from build123d import *

# Parameters (mm, degrees)
F0_W     = 46
F0_H     = 43
F0_R     = 2.5
F1_DEPTH = 3.5
F2_R     = 0.5


with BuildPart() as f1:
    # F0 (on Top) → F1 (new body)
    with BuildSketch(Plane.XY):
        with Locations((-3.022213, -8.843659)):
            Rectangle(F0_W, F0_H)
        with Locations((-3.022213, -12.343659)):
            Circle(F0_R, mode=Mode.SUBTRACT)
    extrude(amount=F1_DEPTH)

    # F2
    f2_edges = [f1.edges().sort_by_distance(p)[0] for p in [
        (-3.022213, 12.656341, 3.5),
        (-26.022213, -8.843659, 3.5),
        (-3.022213, -30.343659, 3.5),
        (19.977787, -8.843659, 3.5),
        (-5.522213, -12.343659, 3.5),
    ]]
    fillet(f2_edges, radius=F2_R)


solid = f1.part
Verification items for the finished model (mm, model axes). Give positions to 0.01 mm unless a question says otherwise; leave off trailing zeros.
1) Thickness scan on line 1 along Y through (x, z) = (-5, 3.3); line 2 along X through (y, z) = (-13.5, 2.9); line 3 along X through (y, z) = (-14.5, 2). Record the ranges inside material, lowest first.
2) Depth check by flat-ended pin: pin 1 Ø8 at (x, y) = (-9, -12.5) entering from -Z. Enter the tip coordinate at first touch or a pass-through.
3) Draft check along X on faces 1 (the flat face through (-3, -9, 0)), 2 (the cylindrical face through (-3.564, -14.784, 1.479)), 3 (the flat face through (-26.022, -9, 1)). Enter one of: pulls with the +X half, pulls with the -X half, needs draft (parallel to the pull), parting line crosses it, or undercut.
Answers:
1. line 1: y = -30.24 to -14.03, -10.66 to 12.56
1. line 2: x = -26.02 to -5.24, -0.81 to 19.98
1. line 3: x = -26.02 to -4.29, -1.76 to 19.98
2. pin 1: stops at z = 0
3. face 1: needs draft
3. face 2: undercut
3. face 3: pulls with the -X half
